Here's how the part is built. I have some questions about the finished solid (model axes, mm). A direction names the side the tool comes from. Give positions to 0.01 mm unless a question says otherwise; leave off trailing zeros. Loops run counter-clockwise (first coordinate to the right, second up) from the corner with the lowest first, then second, coordinate; pieces in that order, holes last.
Q1. Suppose I cut it at B-B (x = 25.4). List the corners of the cut face in (y, z) for me (3 decimals).
Q2. Thinking about a two-plate mould opening in Y: for faces 3 (the face through (21, 0, 216)), 4 (the face through (23.727, 1.565, 409.476)), 5 (the face through (1.61, 16.61, 107.09)), which applies, pulls with the +Y half, pulls with the -Y half, needs draft (parallel to the pull), parting line crosses it, or undercut?
Q3. Suppose I cut it at A-A (z = 25.4). List the corners of the cut face in (x, y) for me (3 decimals).
Q4. For faces 1 (the face through (47.625, 22, 216)), 2 (the face through (49.235, 14.023, 328.734)), which set-ups out of +Z, -Z, +X, -X, +Y, -Y let a thin tool reach every point of the face, with its end or its side?
Q5. I need wall thicknesses on probe 1 along X at (y, z) = (7.5, 296) (3 decimals); probe 2 along Y at (x, z) = (40.5, 180) (3 decimals); probe 3 along X at (y, z) = (3, 22). Which ranges of each line are inside material? Lowest first, please.
Q6. Suppose I cut it at C-C (z = 137). List the corners of the cut face in (x, y) for me (3 decimals).
```python
from build123d import *

# Parameters (mm, degrees)
BASE_FLANGE1_DEPTH = 438.912
SKETCH6_R          = 2.4257
CUT_EXTRUDE1_DEPTH = 444.481672388
SKETCH7_R          = 4.3688
CUT_EXTRUDE2_DEPTH = 444.481672388
SKETCH8_R          = 4.3688
CUT_EXTRUDE3_DEPTH = 444.481672388
FILLET1_R          = 3.175


# Sheet-metal steps are written as plain solids
with BuildPart() as part:
    # Sketch1 → Base-Flange1 (new body)
    with BuildSketch(Plane.XY):
        with BuildLine():
            Line((50.8, 38.1), (50.8, 6.35))
            ThreePointArc((50.8, 6.35), (48.940128061, 1.859871939), (44.45, 0))
            Line((44.45, 0), (6.35, 0))
            ThreePointArc((6.35, 0), (1.859871939, 1.859871939), (0, 6.35))
            Line((0, 6.35), (0, 38.1))
            Line((0, 38.1), (3.175, 38.1))
            Line((3.175, 38.1), (3.175, 6.35))
            ThreePointArc((3.175, 6.35), (4.10493597, 4.10493597), (6.35, 3.175))
            Line((6.35, 3.175), (44.45, 3.175))
            ThreePointArc((44.45, 3.175), (46.69506403, 4.10493597), (47.625, 6.35))
            Line((47.625, 6.35), (47.625, 38.1))
            Line((47.625, 38.1), (50.8, 38.1))
        make_face()
    extrude(amount=BASE_FLANGE1_DEPTH)

    # Sketch6 → Cut-Extrude1 (cut, through all)
    with BuildSketch(Plane(origin=(50.8, 0, 0), x_dir=(0, 0, -1), z_dir=(1, 0, 0))):
        with Locations((-15.875, 15.875)):
            Circle(SKETCH6_R)
        with Locations((-41.275, 15.875)):
            Circle(SKETCH6_R)
        with Locations((-66.675, 15.875)):
            Circle(SKETCH6_R)
        with Locations((-372.237, 15.875)):
            Circle(SKETCH6_R)
        with Locations((-397.637, 15.875)):
            Circle(SKETCH6_R)
        with Locations((-423.037, 15.875)):
            Circle(SKETCH6_R)
        with Locations((-92.075, 15.875)):
            Circle(SKETCH6_R)
        with Locations((-346.837, 15.875)):
            Circle(SKETCH6_R)
    extrude(amount=-CUT_EXTRUDE1_DEPTH, mode=Mode.SUBTRACT)

    # Sketch7 → Cut-Extrude2 (cut, through all)
    with BuildSketch(Plane.XZ):
        with Locations(Location((25.4, 219.456, 0), (0, 0, 270))):
            Circle(SKETCH7_R)
        with Locations(Location((25.4, 25.4, 0), (0, 0, 270))):
            Circle(SKETCH7_R)
        with Locations(Location((25.4, 413.512, 0), (0, 0, 270))):
            Circle(SKETCH7_R)
    extrude(amount=-CUT_EXTRUDE2_DEPTH, mode=Mode.SUBTRACT)

    # Sketch8 → Cut-Extrude3 (cut, through all)
    with BuildSketch(Plane(origin=(50.8, 0, 0), x_dir=(0, 0, -1), z_dir=(1, 0, 0))):
        with Locations((-111.125, 18.288)):
            Circle(SKETCH8_R)
        with Locations((-327.787, 18.288)):
            Circle(SKETCH8_R)
    extrude(amount=-CUT_EXTRUDE3_DEPTH, mode=Mode.SUBTRACT)

    # Fillet1
    fillet1_edges = [part.edges().sort_by_distance(p)[0] for p in [
        (1.5875, 38.1, 0),
        (49.2125, 38.1, 0),
        (1.5875, 38.1, 438.912),
        (49.2125, 38.1, 438.912),
    ]]
    fillet(fillet1_edges, radius=FILLET1_R)


solid = part.part
```
Solutions:
1. outline: (0, 0) - (3.175, 0) - (3.175, 21.031) - (0, 21.031) - close; (0, 29.769) - (3.175, 29.769) - (3.175, 215.087) - (0, 215.087) - close; (0, 223.825) - (3.175, 223.825) - (3.175, 409.143) - (0, 409.143) - close; (0, 417.881) - (3.175, 417.881) - (3.175, 438.912) - (0, 438.912) - close
2. face 3: pulls with the -Y half
2. face 4: needs draft
2. face 5: undercut
3. outline: (0, 6.35) arc R6.35 ccw to (6.35, 0) - (21.031, 0) - (21.031, 3.175) - (6.35, 3.175) arc R3.175 cw to (3.175, 6.35) - (3.175, 38.1) - (0, 38.1) - close; (29.769, 0) - (44.45, 0) arc R6.35 ccw to (50.8, 6.35) - (50.8, 38.1) - (47.625, 38.1) - (47.625, 6.35) arc R3.175 cw to (44.45, 3.175) - (29.769, 3.175) - close
4. face 1: +Z, -Z, +Y
4. face 2: +X, -X
5. probe 1: x = 0 to 3.175, 47.625 to 50.8
5. probe 2: y = 0 to 3.175
5. probe 3: x = 0.96 to 22.66, 28.14 to 49.84
6. outline: (0, 6.35) arc R6.35 ccw to (6.35, 0) - (44.45, 0) arc R6.35 ccw to (50.8, 6.35) - (50.8, 38.1) - (47.625, 38.1) - (47.625, 6.35) arc R3.175 cw to (44.45, 3.175) - (6.35, 3.175) arc R3.175 cw to (3.175, 6.35) - (3.175, 38.1) - (0, 38.1) - close
